Here's the drawing with two shaded views (mm, measured from the low corner). I have some questions. Give positions to 0.01 mm unless a question says otherwise; leave off trailing zeros. Write each loop counter-clockwise with the first axis right and the second up, starting at its lowest first coordinate (ties: lowest second). Pieces come first, ordered by that corner, then holes. Notation, with made-up numbers: (-40, 61.5) -> (14, 61.5) arc R32 cw to (14, 88.5) -> close; hole circle Ø2 at (80, -28.5). An arc over 180 degrees is marked (long way). Put each result on its own line as item: value. Start each with the question number.
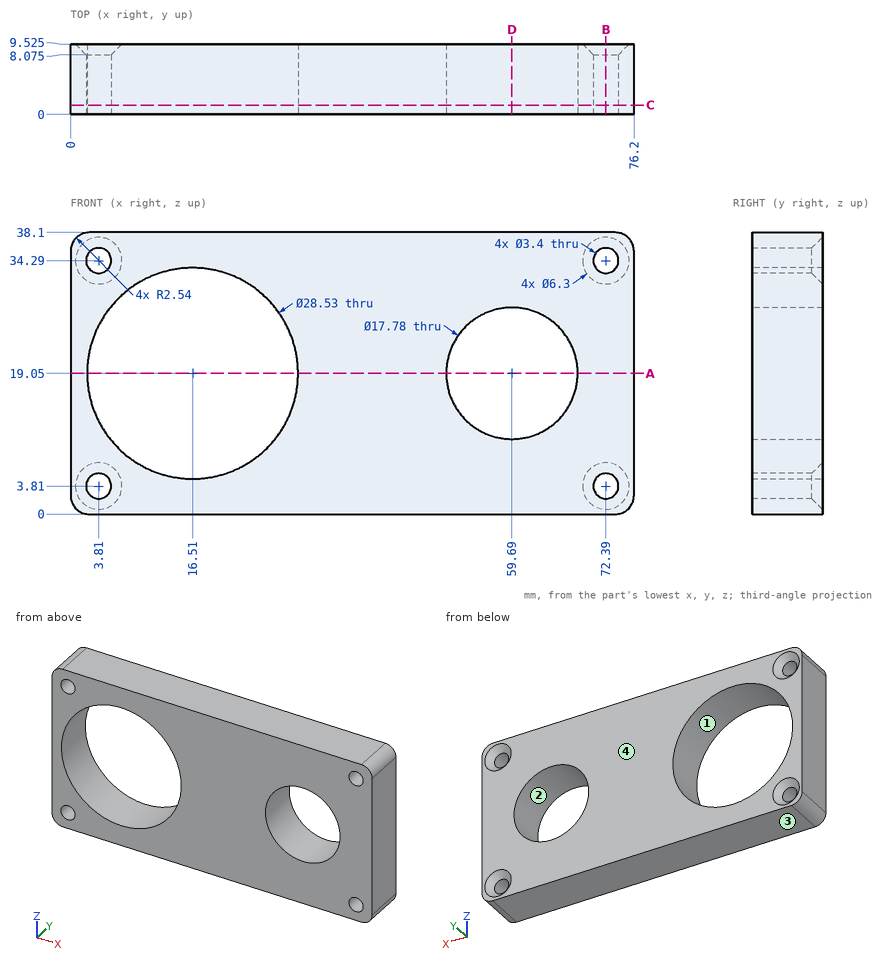
1) I'm going to push flat-ended pins straight in: pin 1 Ø4.5 at (x, z) = (72.39, 3.81) entering from +Y (3 decimals); pin 2 Ø2 at (x, z) = (72.39, 34.29) entering from -Y; pin 3 Ø5.5 at (x, z) = (3.81, 34.29) entering from +Y (3 decimals). Where does each tip first touch, or does it pass through?
2) Thinking about a two-plate mould opening in Z: for the marked faces 1, 2, 3 and 4, which applies, released by +Z, released by -Z, zero draft, split by the parting line, or undercut?
3) I want a section at A-A, the plane z = 19.05. Write out the boundary of the cut face in (x, y) (3 decimals).
4) I need wall thicknesses on probe 1 along X at (y, z) = (3.75, 19.05) (3 decimals); probe 2 along X at (y, z) = (2, 34.29); probe 3 along Z at (x, y) = (21, 3.75). Which ranges of each line are inside material? Lowest first, please.
5) I want a section at B-B, the plane x = 72.39. Write out the boundary of the cut face in (y, z) (3 decimals).
6) I want a section at C-C, the plane y = 1.25. Write out the boundary of the cut face in (x, z) (3 decimals).
7) I want a section at D-D, the plane x = 59.69. Write out the boundary of the cut face in (y, z) (3 decimals), and give its area (3 significant figures).
Established:
1. pin 1: stops at y = 8.625
1. pin 2: passes through
1. pin 3: stops at y = 9.125
2. face 1: undercut
2. face 2: undercut
2. face 3: released by -Z
2. face 4: zero draft
3. outline: (0, 0) -> (2.245, 0) -> (2.245, 9.525) -> (0, 9.525) -> close; (30.775, 0) -> (50.8, 0) -> (50.8, 9.525) -> (30.775, 9.525) -> close; (68.58, 0) -> (76.2, 0) -> (76.2, 9.525) -> (68.58, 9.525) -> close
4. probe 1: x = 0 to 2.245, 30.775 to 50.8, 68.58 to 76.2
4. probe 2: x = 0 to 2.11, 5.51 to 70.69, 74.09 to 76.2
4. probe 3: z = 0 to 5.51, 32.59 to 38.1
5. outline: (0, 0) -> (9.525, 0) -> (9.525, 0.66) -> (8.075, 2.11) -> (0, 2.11) -> close; (0, 5.51) -> (8.075, 5.51) -> (9.525, 6.96) -> (9.525, 31.14) -> (8.075, 32.59) -> (0, 32.59) -> close; (0, 35.99) -> (8.075, 35.99) -> (9.525, 37.44) -> (9.525, 38.1) -> (0, 38.1) -> close
6. outline: (0, 2.54) arc R2.54 ccw to (2.54, 0) -> (73.66, 0) arc R2.54 ccw to (76.2, 2.54) -> (76.2, 35.56) arc R2.54 ccw to (73.66, 38.1) -> (2.54, 38.1) arc R2.54 ccw to (0, 35.56) -> close; hole circle Ø3.4 at (3.81, 3.81); hole circle Ø3.4 at (3.81, 34.29); hole circle Ø28.53 at (16.51, 19.05); hole circle Ø17.78 at (59.69, 19.05); hole circle Ø3.4 at (72.39, 3.81); hole circle Ø3.4 at (72.39, 34.29)
7. outline: (0, 0) -> (9.525, 0) -> (9.525, 10.16) -> (0, 10.16) -> close; (0, 27.94) -> (9.525, 27.94) -> (9.525, 38.1) -> (0, 38.1) -> close
7. area: 194 mm2
